from build123d import *

# Parameters (mm, degrees)
EXTRUDE_1_DEPTH = 4


with BuildPart() as part:
    # 草图1 → 凸台-拉伸1 (new, symmetric)
    with BuildSketch(Plane.XY):
        with BuildLine():
            Line((-692.368123223, 756.238006891), (-692.368123223, 714.238006891))
            Line((-692.368123223, 714.238006891), (-812.368123223, 714.238006891))
            ThreePointArc((-812.368123223, 714.238006891), (-878.129053873, 741.477076241), (-905.368123223, 807.238006891))
            Line((-905.368123223, 807.238006891), (-905.368123223, 851.650469452))
            Line((-905.368123223, 851.650469452), (-865.837171529, 884.820876438))
            ThreePointArc((-865.837171529, 884.820876438), (-852.397642484, 902.335611688), (-847.619339623, 923.889143037))
            Line((-847.619339623, 923.889143037), (-847.619339623, 1124.889143037))
            Line((-847.619339623, 1124.889143037), (-796.619339623, 1124.889143037))
            ThreePointArc((-796.619339623, 1124.889143037), (-727.873290815, 1112.767359815), (-667.419030076, 1077.864076104))
            Line((-667.419030076, 1077.864076104), (-515.368123223, 898.238006891))
            Line((-515.368123223, 898.238006891), (-515.368123223, 858.238006891))
            Line((-515.368123223, 858.238006891), (-812.368123223, 858.238006891))
            ThreePointArc((-812.368123223, 858.238006891), (-863.368123223, 807.238006891), (-812.368123223, 756.238006891))
            Line((-812.368123223, 756.238006891), (-692.368123223, 756.238006891))
        make_face()
    extrude(amount=EXTRUDE_1_DEPTH, both=True)


solid = part.part
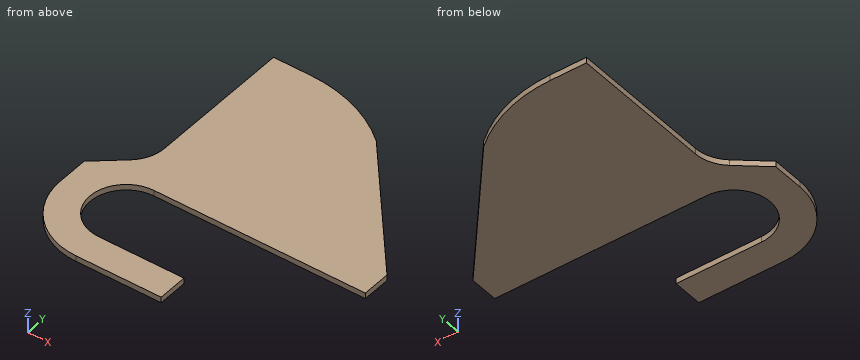
Geometry: final body of the model. Coordinates: model frame, mm. Round coordinates to 2 decimals unless told otherwise and drop trailing zeros. Loops run counter-clockwise (first coordinate to the right, second up) from the corner with the lowest first, then second, coordinate; pieces in that order, holes last. Notation, with made-up numbers: (88.25, 8.25) -> (136.25, 8.25) arc R24 ccw to (136.25, 40.25) -> close; hole circle Ø2 at (11.5, 55.5). An arc over 180 degrees is marked (long way). One line per question, with ' | ' between items. Start each with the question number.
1. Line query: line 1 along Y through (x, z) = (-790.5, 2.5); line 2 along Y through (x, z) = (-788.5, -2.75); line 3 along X through (y, z) = (773, 2.5). Output: solid intervals per line, ascending. Write a range as [from, to].
2. Section C-C on x = -698. Output: boundary loops of the cut face in (y, z).
3. Contact query for flat-ended pins moving along their axis: pin 1 (1 mm diameter, centred on y = 930, z = -1.5, fed in from +X); pin 2 (2.5 mm diameter, centred on y = 743.5, z = 0, fed in from +X); pin 3 (2 mm diameter, centred on y = 852, z = -2.5, fed in from +X). Output: stop coordinate, or through.
4. Section D-D on y = 1070. Output: boundary loops of the cut face in (x, z).
5. Section A-A on x = -753. Output: boundary loops of the cut face in (y, z), and give its area (3 significant figures).
6. Section B-B on z = 0. Output: boundary loops of the cut face in (x, y).
Returned:
1) line 1: y = [714.24, 756.24], [858.24, 1124.8] | line 2: y = [714.24, 756.24], [858.24, 1124.73] | line 3: x = [-898.84, -850.17]
2) outline: (714.24, -4) -> (756.24, -4) -> (756.24, 4) -> (714.24, 4) -> close; (858.24, -4) -> (1099.03, -4) -> (1099.03, 4) -> (858.24, 4) -> close
3) pin 1: stops at x = -541.83 | pin 2: stops at x = -692.37 | pin 3: stops at x = -834.88
4) outline: (-847.62, -4) -> (-660.76, -4) -> (-660.76, 4) -> (-847.62, 4) -> close
5) outline: (714.24, -4) -> (756.24, -4) -> (756.24, 4) -> (714.24, 4) -> close; (858.24, -4) -> (1120.1, -4) -> (1120.1, 4) -> (858.24, 4) -> close | area: 2,430 mm2
6) outline: (-905.37, 807.24) arc R93 ccw to (-812.37, 714.24) -> (-692.37, 714.24) -> (-692.37, 756.24) -> (-812.37, 756.24) arc R51 cw to (-812.37, 858.24) -> (-515.37, 858.24) -> (-515.37, 898.24) -> (-667.42, 1077.86) arc R201 ccw to (-796.62, 1124.89) -> (-847.62, 1124.89) -> (-847.62, 923.89) arc R51 cw to (-865.84, 884.82) -> (-905.37, 851.65) -> close
